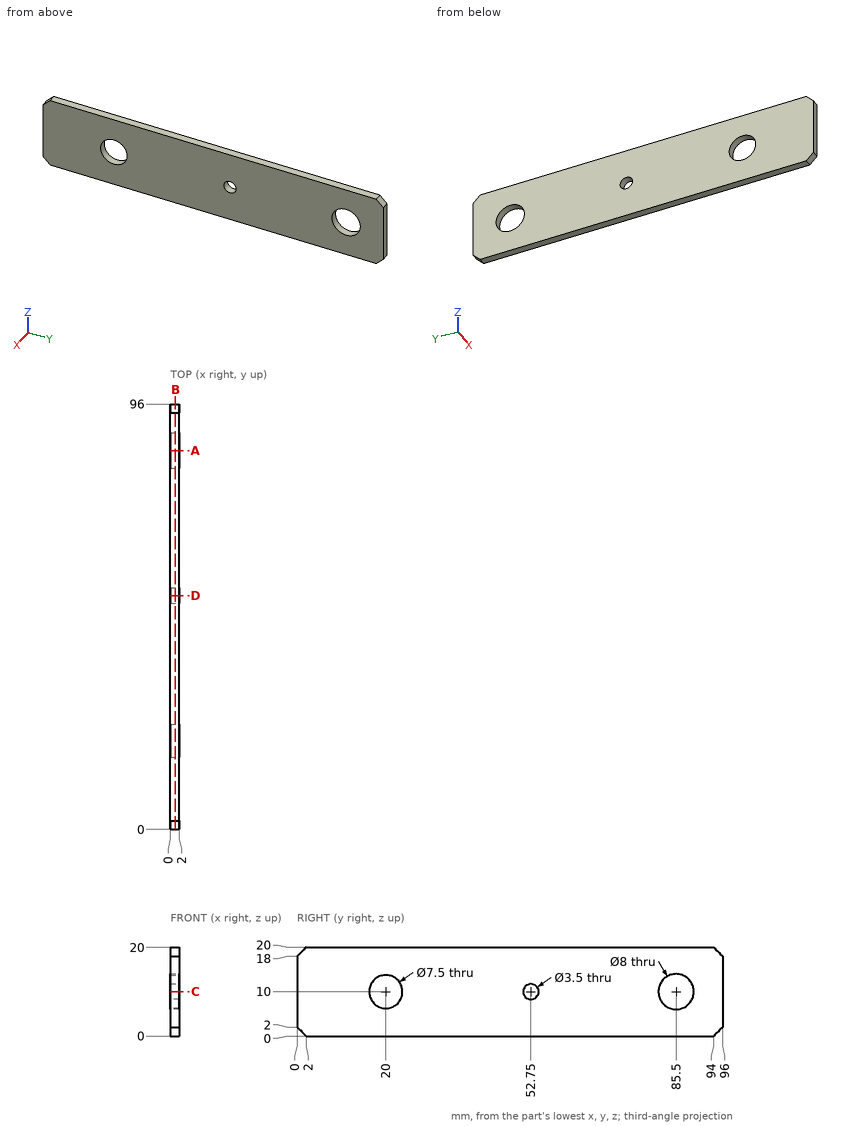
Drawing for the job (mm, zero at the part's lowest x, y, z). Give positions to 0.01 mm unless a question says otherwise; leave off trailing zeros. Write each loop counter-clockwise with the first axis right and the second up, starting at its lowest first coordinate (ties: lowest second). Pieces come first, ordered by that corner, then holes. Notation, with made-up numbers: (-12, -15) -> (-7, -15) arc R26 cw to (-7, 4) -> close; hole circle Ø3 at (-17, -8). An arc over 180 degrees is marked (long way). Put each result on its own line as item: value. Start each with the question number.
Item 1: Cut at D-D (y = 52.75). List the corners of the cut face in (x, z), then the cut area to 3 significant figures.
Item 2: Wall check: L1, parallel to Y at x = 1.45, z = 10; L2, parallel to Y at x = 0.6, z = 9; L3, parallel to Y at x = 1.5, z = 18.25. Give the ranges that are in metal, low to high. Write a range as [from, to].
Item 3: Cut at B-B (x = 1.1). List the corners of the cut face in (y, z).
Item 4: Cut at C-C (z = 10). List the corners of the cut face in (x, y), then the cut area to 3 significant figures.
Item 5: Cut at A-A (y = 85.5). List the corners of the cut face in (x, z).
Item 6: Pin check, flat tips, straight feed: pin 1 Ø4 at (y, z) = (69, 14.5) entering from -X; pin 2 Ø4.5 at (y, z) = (20, 10) entering from -X. Stop position of each tip, or through.
Answer list:
1. outline: (0, 0) -> (2, 0) -> (2, 8.25) -> (0, 8.25) -> close; (0, 11.75) -> (2, 11.75) -> (2, 20) -> (0, 20) -> close
1. area: 33.0 mm2
2. L1: y = [0, 16.25], [23.75, 51], [54.5, 81.5], [89.5, 96]
2. L2: y = [0, 16.39], [23.61, 51.31], [54.19, 81.63], [89.37, 96]
2. L3: y = [0.25, 95.75]
3. outline: (0, 2) -> (2, 0) -> (94, 0) -> (96, 2) -> (96, 18) -> (94, 20) -> (2, 20) -> (0, 18) -> close; hole circle Ø7.5 at (20, 10); hole circle Ø3.5 at (52.75, 10); hole circle Ø8 at (85.5, 10)
4. outline: (0, 0) -> (2, 0) -> (2, 16.25) -> (0, 16.25) -> close; (0, 23.75) -> (2, 23.75) -> (2, 51) -> (0, 51) -> close; (0, 54.5) -> (2, 54.5) -> (2, 81.5) -> (0, 81.5) -> close; (0, 89.5) -> (2, 89.5) -> (2, 96) -> (0, 96) -> close
4. area: 154 mm2
5. outline: (0, 0) -> (2, 0) -> (2, 6) -> (0, 6) -> close; (0, 14) -> (2, 14) -> (2, 20) -> (0, 20) -> close
6. pin 1: stops at x = 0
6. pin 2: passes through
